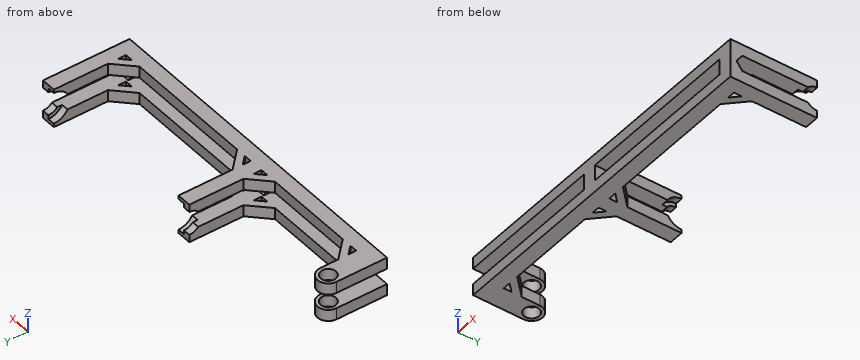
```python
from build123d import *

# Parameters (mm, degrees)
SKETCH1_R               = 5.25
BOSS_EXTRUDE1_DEPTH     = 8
BOSS_EXTRUDE2_DEPTH     = 10
LPATTERN1_COUNT         = 2
LPATTERN1_PITCH         = 125
MIRROR1_COPY_1_DEPTH    = 10
CUT_EXTRUDE1_START      = -5
SKETCH3_R               = 11
CUT_EXTRUDE1_DEPTH      = 125
CUT_EXTRUDE2_DEPTH      = 10
CUT_EXTRUDE2_DEPTH_BACK = 149.949655924
SKETCH4_R               = 8.25


with BuildPart() as part:
    # Sketch1 → Boss-Extrude1 (new body)
    with BuildSketch(Plane.XY):
        with BuildLine():
            Line((230, 0), (230, 60))
            Line((230, 60), (220, 60))
            Line((220, 60), (220, 22.5))
            Line((220, 22.5), (207.5, 10))
            Line((207.5, 10), (117.5, 10))
            Line((117.5, 10), (105, 22.5))
            Line((105, 22.5), (105, 60))
            Line((105, 60), (95, 60))
            Line((95, 60), (95, 22.5))
            Line((95, 22.5), (82.5, 10))
            Line((82.5, 10), (20, 10))
            Line((20, 10), (7.5, 22.5))
            Line((7.5, 22.5), (7.5, 35))
            ThreePointArc((7.5, 35), (0, 42.5), (-7.5, 35))
            Line((-7.5, 35), (-7.5, 0))
            Line((-7.5, 0), (230, 0))
        make_face()
        Polygon((95, 15.428932188), (95, 10), (89.571067812, 10), align=None, mode=Mode.SUBTRACT)
        Polygon((110.428932188, 10), (105, 10), (105, 15.428932188), align=None, mode=Mode.SUBTRACT)
        Polygon((220, 15.428932188), (220, 10), (214.571067812, 10), align=None, mode=Mode.SUBTRACT)
        with Locations((0, 35)):
            Circle(SKETCH1_R, mode=Mode.SUBTRACT)
        Polygon((7.5, 15.428932188), (12.928932188, 10), (7.5, 10), align=None, mode=Mode.SUBTRACT)
    boss_extrude1 = extrude(amount=BOSS_EXTRUDE1_DEPTH)

    # Sketch2 → Boss-Extrude2 (add)
    with BuildSketch(Plane(origin=(95, 0, 0), x_dir=(0, 0, -1), z_dir=(1, 0, 0))):
        Polygon((5.5, 4.166666667), (0, 8.333333333), (0, 0), (5.5, 0), align=None)
    boss_extrude2 = extrude(amount=BOSS_EXTRUDE2_DEPTH)

    # LPattern1: Boss-Extrude2 ×2
    with Locations(*[(i * LPATTERN1_PITCH, 0, 0) for i in range(1, LPATTERN1_COUNT)]):
        add(boss_extrude2)

    # Mirror1: Boss-Extrude1, Boss-Extrude2 across plane
    add(boss_extrude1.mirror(Plane(origin=(105, 0, -5.5), x_dir=(1, 0, 0), z_dir=(0, 0, 1))))
    add(boss_extrude2.mirror(Plane(origin=(105, 0, -5.5), x_dir=(1, 0, 0), z_dir=(0, 0, 1))))

    # Mirror1 copy 1 sketch → Mirror1 copy 1 (add)
    with BuildSketch(Plane(origin=(220, 0, -11), x_dir=(0, 0, 1), z_dir=(1, 0, 0))):
        Polygon((5.5, -4.166666667), (0, -8.333333333), (0, 0), (5.5, 0), align=None)
    extrude(amount=MIRROR1_COPY_1_DEPTH)

    # Sketch3 → Cut-Extrude1 (cut)
    with BuildSketch(Plane(origin=(105, 0, 0), x_dir=(0, 0, -1), z_dir=(1, 0, 0)).offset(CUT_EXTRUDE1_START)):
        with Locations((5.5, 60)):
            Circle(SKETCH3_R)
    extrude(amount=CUT_EXTRUDE1_DEPTH, mode=Mode.SUBTRACT)

    # Sketch4 → Cut-Extrude2 (cut, two sides: drawn at the far end of the back side and taken through both)
    with BuildSketch(Plane.ZY.offset(-95).offset(-CUT_EXTRUDE2_DEPTH_BACK)):
        with Locations((-5.5, 60)):
            Circle(SKETCH4_R)
    extrude(amount=CUT_EXTRUDE2_DEPTH + CUT_EXTRUDE2_DEPTH_BACK, mode=Mode.SUBTRACT)


solid = part.part
```
Source: CAD feature listing. Evaluate the final solid. Frame: model axes, mm. Coordinates: 2 decimals unless noted, no trailing zeros. Write each loop counter-clockwise with the first axis right and the second up, starting at its lowest first coordinate (ties: lowest second). Pieces come first, ordered by that corner, then holes. Notation, with made-up numbers: (25.25, 78.25) -> (80.25, 78.25) arc R29 cw to (80.25, 98.25) -> close; hole circle Ø9 at (30.25, 76.25). An arc over 180 degrees is marked (long way). Return JSON: item names as keys, results as strings. Group by question number.
1) Section query A-A, the plane x = 209.5. Return loops of the section in (y, z), plus the area to 3 significant figures.
2) Section query C-C, the plane x = 151.5. Return loops of the section in (y, z).
3) Section query B-B, the plane x = 0. Return loops of the section in (y, z).
4) Contact query for flat-ended pins moving along their axis: P1, Ø6.5, axis at x = 143.5, z = 5.5, coming from the +Y side; P2, Ø6, axis at y = 56, z = 2.5, coming from the -X side; P3, Ø4, axis at y = 36.5, z = -11.5, coming from the -X side; P4, Ø2.5, axis at x = 10.5, z = -13, coming from the +Y side. Output: stop coordinate, or through.
5) Ray query, line 1 along Y through (x, z) = (0, 3.25); line 2 along Z through (x, y) = (122, 8); line 3 along X through (y, z) = (4.5, -1). Return the intervals inside material, ascending.
From the geometry:
{
 "1": {"outline": "(0, -19) -> (12, -19) -> (12, -11) -> (0, -11) -> close; (0, 0) -> (12, 0) -> (12, 8) -> (0, 8) -> close", "area": "192 mm²"},
 "2": {"outline": "(0, -19) -> (10, -19) -> (10, -11) -> (0, -11) -> close; (0, 0) -> (10, 0) -> (10, 8) -> (0, 8) -> close"},
 "3": {"outline": "(0, -19) -> (29.75, -19) -> (29.75, -11) -> (0, -11) -> close; (0, 0) -> (29.75, 0) -> (29.75, 8) -> (0, 8) -> close; (40.25, -19) -> (42.5, -19) -> (42.5, -11) -> (40.25, -11) -> close; (40.25, 0) -> (42.5, 0) -> (42.5, 8) -> (40.25, 8) -> close"},
 "4": {"P1": "y = 10", "P2": "x = 95", "P3": "x = -7.5", "P4": "y = 20.75"},
 "5": {"line 1": "0 to 29.75, 40.25 to 42.5", "line 2": "-19 to -11, 0 to 8", "line 3": "95 to 105, 220 to 230"}
}
